from build123d import *

# Parameters (mm, degrees)
SKETCH1_R           = 65
SKETCH1_R_2         = 55
BOSS_EXTRUDE1_DEPTH = 250
BOSS_EXTRUDE2_START = 20
SKETCH3_R           = 55
SKETCH3_R_2         = 20
SKETCH3_R_3         = 13
BOSS_EXTRUDE2_DEPTH = 20
BOSS_EXTRUDE3_START = 210
SKETCH3_5_R         = 55
SKETCH3_5_R_2       = 20
SKETCH3_5_R_3       = 13
SKETCH3_5_R_4       = 6.5
BOSS_EXTRUDE3_DEPTH = 20
BOSS_EXTRUDE4_START = 20
SKETCH3_7_R         = 13
BOSS_EXTRUDE4_DEPTH = 210
SKETCH3_10_R        = 13
BOSS_EXTRUDE5_DEPTH = 20
BOSS_EXTRUDE6_START = 230
SKETCH3_11_R        = 13
BOSS_EXTRUDE6_DEPTH = 20


with BuildPart() as part:
    # Sketch1 → Boss-Extrude1 (new body)
    with BuildSketch(Plane(origin=(0, 0, 0), x_dir=(1, 0, 0), z_dir=(0, 1, 0))):
        with Locations(Location((0, 0, 0), (0, 0, 270))):
            Circle(SKETCH1_R)
        with Locations(Location((0, 0, 0), (0, 0, 270))):
            Circle(SKETCH1_R_2, mode=Mode.SUBTRACT)
    extrude(amount=BOSS_EXTRUDE1_DEPTH)

    # Sketch3 → Boss-Extrude2 (add)
    with BuildSketch(Plane(origin=(0, 0, 0), x_dir=(1, 0, 0), z_dir=(0, 1, 0)).offset(BOSS_EXTRUDE2_START)):
        with Locations(Location((0, 0, 0), (0, 0, 270))):
            Circle(SKETCH3_R)
        with BuildLine():
            ThreePointArc((39.298819185, 16.181866723), (42.375869887, 3.245866806), (41.304875194, -10.00786117))
            Line((41.304875194, -10.00786117), (19.437588327, -4.709581727))
            ThreePointArc((19.437588327, -4.709581727), (17.030904249, -10.485623513), (12.957116602, -15.235259412))
            Line((12.957116602, -15.235259412), (27.53387278, -32.374926251))
            ThreePointArc((27.53387278, -32.374926251), (16.181866723, -39.298819185), (3.245866806, -42.375869887))
            Line((3.245866806, -42.375869887), (1.527466732, -19.941585829))
            ThreePointArc((1.527466732, -19.941585829), (-4.709581727, -19.437588327), (-10.485623513, -17.030904249))
            Line((-10.485623513, -17.030904249), (-22.281949965, -36.190671529))
            ThreePointArc((-22.281949965, -36.190671529), (-32.374926251, -27.53387278), (-39.298819185, -16.181866723))
            Line((-39.298819185, -16.181866723), (-18.493561969, -7.614996105))
            ThreePointArc((-18.493561969, -7.614996105), (-19.941585829, -1.527466732), (-19.437588327, 4.709581727))
            Line((-19.437588327, 4.709581727), (-41.304875194, 10.00786117))
            ThreePointArc((-41.304875194, 10.00786117), (-36.190671529, 22.281949965), (-27.53387278, 32.374926251))
            Line((-27.53387278, 32.374926251), (-12.957116602, 15.235259412))
            ThreePointArc((-12.957116602, 15.235259412), (-7.614996105, 18.493561969), (-1.527466732, 19.941585829))
            Line((-1.527466732, 19.941585829), (-3.245866806, 42.375869887))
            ThreePointArc((-3.245866806, 42.375869887), (10.00786117, 41.304875194), (22.281949965, 36.190671529))
            Line((22.281949965, 36.190671529), (10.485623513, 17.030904249))
            ThreePointArc((10.485623513, 17.030904249), (15.235259412, 12.957116602), (18.493561969, 7.614996105))
            Line((18.493561969, 7.614996105), (39.298819185, 16.181866723))
        make_face(mode=Mode.SUBTRACT)
        Circle(SKETCH3_R_2)
        with Locations(Location((0, 0, 0), (0, 0, 270))):
            Circle(SKETCH3_R_3, mode=Mode.SUBTRACT)
    extrude(amount=BOSS_EXTRUDE2_DEPTH)

    # Sketch3_5 → Boss-Extrude3 (add)
    with BuildSketch(Plane(origin=(0, 0, 0), x_dir=(1, 0, 0), z_dir=(0, 1, 0)).offset(BOSS_EXTRUDE3_START)):
        with Locations(Location((0, 0, 0), (0, 0, 270))):
            Circle(SKETCH3_5_R)
        with BuildLine():
            ThreePointArc((39.298819185, 16.181866723), (42.375869887, 3.245866806), (41.304875194, -10.00786117))
            Line((41.304875194, -10.00786117), (19.437588327, -4.709581727))
            ThreePointArc((19.437588327, -4.709581727), (17.030904249, -10.485623513), (12.957116602, -15.235259412))
            Line((12.957116602, -15.235259412), (27.53387278, -32.374926251))
            ThreePointArc((27.53387278, -32.374926251), (16.181866723, -39.298819185), (3.245866806, -42.375869887))
            Line((3.245866806, -42.375869887), (1.527466732, -19.941585829))
            ThreePointArc((1.527466732, -19.941585829), (-4.709581727, -19.437588327), (-10.485623513, -17.030904249))
            Line((-10.485623513, -17.030904249), (-22.281949965, -36.190671529))
            ThreePointArc((-22.281949965, -36.190671529), (-32.374926251, -27.53387278), (-39.298819185, -16.181866723))
            Line((-39.298819185, -16.181866723), (-18.493561969, -7.614996105))
            ThreePointArc((-18.493561969, -7.614996105), (-19.941585829, -1.527466732), (-19.437588327, 4.709581727))
            Line((-19.437588327, 4.709581727), (-41.304875194, 10.00786117))
            ThreePointArc((-41.304875194, 10.00786117), (-36.190671529, 22.281949965), (-27.53387278, 32.374926251))
            Line((-27.53387278, 32.374926251), (-12.957116602, 15.235259412))
            ThreePointArc((-12.957116602, 15.235259412), (-7.614996105, 18.493561969), (-1.527466732, 19.941585829))
            Line((-1.527466732, 19.941585829), (-3.245866806, 42.375869887))
            ThreePointArc((-3.245866806, 42.375869887), (10.00786117, 41.304875194), (22.281949965, 36.190671529))
            Line((22.281949965, 36.190671529), (10.485623513, 17.030904249))
            ThreePointArc((10.485623513, 17.030904249), (15.235259412, 12.957116602), (18.493561969, 7.614996105))
            Line((18.493561969, 7.614996105), (39.298819185, 16.181866723))
        make_face(mode=Mode.SUBTRACT)
        Circle(SKETCH3_5_R_2)
        with Locations(Location((0, 0, 0), (0, 0, 270))):
            Circle(SKETCH3_5_R_3, mode=Mode.SUBTRACT)
        Circle(SKETCH3_5_R_4)
    extrude(amount=BOSS_EXTRUDE3_DEPTH)


with BuildPart() as boss_extrude3_kept_piece:
    # of the separate pieces the step leaves, the one the design keeps (boss_extrude3_pieces_kept)
    add(part.part.solids().sort_by_distance((0, 0, 65))[0])

    # Sketch3_7 → Boss-Extrude4 (add)
    with BuildSketch(Plane(origin=(0, 0, 0), x_dir=(1, 0, 0), z_dir=(0, 1, 0)).offset(BOSS_EXTRUDE4_START)):
        with Locations(Location((0, 0, 0), (0, 0, 270))):
            Circle(SKETCH3_7_R)
        with BuildLine():
            Line((2, 8.5), (2, 6.184658438))
            ThreePointArc((2, 6.184658438), (5.25594901, 3.824264635), (6.5, 0))
            ThreePointArc((6.5, 0), (-3.824264635, -5.25594901), (-2, 6.184658438))
            Line((-2, 6.184658438), (-2, 8.5))
            Line((-2, 8.5), (2, 8.5))
        make_face(mode=Mode.SUBTRACT)
        with BuildLine():
            ThreePointArc((-2, 6.184658438), (0, 6.5), (2, 6.184658438))
            Line((2, 6.184658438), (2, 8.5))
            Line((2, 8.5), (-2, 8.5))
            Line((-2, 8.5), (-2, 6.184658438))
        make_face()
    extrude(amount=BOSS_EXTRUDE4_DEPTH)

    # Sketch3_10 → Boss-Extrude5 (add)
    with BuildSketch(Plane(origin=(0, 0, 0), x_dir=(1, 0, 0), z_dir=(0, 1, 0))):
        with Locations(Location((0, 0, 0), (0, 0, 270))):
            Circle(SKETCH3_10_R)
        with BuildLine():
            Line((2, 5.656854249), (2, 8.5))
            Line((2, 8.5), (-2, 8.5))
            Line((-2, 8.5), (-2, 5.656854249))
            ThreePointArc((-2, 5.656854249), (0, -6), (2, 5.656854249))
        make_face(mode=Mode.SUBTRACT)
    extrude(amount=BOSS_EXTRUDE5_DEPTH)

    # Sketch3_11 → Boss-Extrude6 (add)
    with BuildSketch(Plane(origin=(0, 0, 0), x_dir=(1, 0, 0), z_dir=(0, 1, 0)).offset(BOSS_EXTRUDE6_START)):
        with Locations(Location((0, 0, 0), (0, 0, 270))):
            Circle(SKETCH3_11_R)
        with BuildLine():
            Line((2, 5.656854249), (2, 8.5))
            Line((2, 8.5), (-2, 8.5))
            Line((-2, 8.5), (-2, 5.656854249))
            ThreePointArc((-2, 5.656854249), (0, -6), (2, 5.656854249))
        make_face(mode=Mode.SUBTRACT)
    extrude(amount=BOSS_EXTRUDE6_DEPTH)


solid = boss_extrude3_kept_piece.part
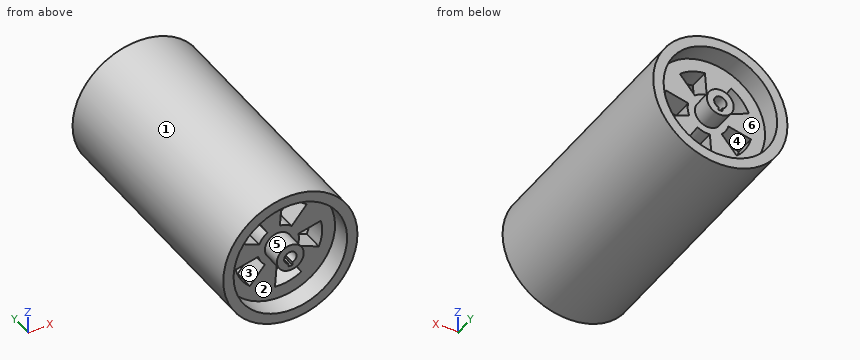
Model file for the job. Use its own axes, mm. Face numbers are marked on the shaded views. A direction names the side the tool comes from. Give positions to 0.01 mm unless a question says otherwise; leave off trailing zeros. Write each loop counter-clockwise with the first axis right and the second up, starting at its lowest first coordinate (ties: lowest second). Pieces come first, ordered by that corner, then holes. Notation, with made-up numbers: M 75,-18.5 L 130,-18.5 A23 ccw 130,7.5 Z; hole C -12.5,28.25 d10. An arc over 180 degrees is marked long. One line per item, written item: value. Start each with the question number.
Q1. Saw through at A-A, the plane y = 217.5. Write the cut outline in (x, z) (3 decimals), plus the area to 3 significant figures.
Q2. Probe probe 1 along X at (y, z) = (19, 0); probe 2 along Y at (x, z) = (39, -35.5); probe 3 along X at (y, z) = (146.5, 4.5). List the from-to ranges inside material, lowest first. Write a range as [from, to].
Q3. Saw through at B-B, the plane z = -23. State how many separate pieces and enclosed holes the cut face has, plus the area to 3 significant figures.
Q4. Drop flat-ended pins along their axis: pin 1 Ø3 at (y, z) = (238.5, -7.5) entering from -X; pin 2 Ø4 at (y, z) = (42, 25) entering from +X; pin 3 Ø2 at (x, y) = (-0.5, 235.5) entering from +Z; pin 4 Ø1 at (x, z) = (-20, 4.5) entering from -Y. Give the stop position or say it passes through.
Q5. Saw through at C-C, the plane y = 147. Write the cut outline in (x, z).
Q6. 3-axis set-ups, long thin cutter, end or side, ignore diameter. For the marked faces 4, 5 and 6: which of +Z, -Z, +X, -X, +Y, -Y reach the whole face in a straight line?
Q7. Two-plate mould, pull along X, no slides. Class the marked faces 1, 2 and 3: +X half, -X half, draft (parallel to the pull), parting line (faces both ways), or undercut.
Output values:
1. outline: C 0,0 d130; hole M -41.305,-10.008 A42.5 ccw -27.534,-32.375 L -12.957,-15.235 A20 cw -19.438,-4.71 Z; hole M -39.299,16.182 L -18.494,7.615 A20 cw -10.486,17.031 L -22.282,36.191 A42.5 ccw Z; hole C 0,0 d13; hole M -3.246,-42.376 A42.5 ccw 22.282,-36.191 L 10.486,-17.031 A20 cw -1.527,-19.942 Z; hole M 1.527,19.942 A20 cw 12.957,15.235 L 27.534,32.375 A42.5 ccw 3.246,42.376 Z; hole M 18.494,-7.615 L 39.299,-16.182 A42.5 ccw 41.305,10.008 L 19.438,4.71 A20 cw Z
1. area: 10,900 mm²
2. probe 1: x = [-65, -55], [-13, -6], [6, 13], [55, 65]
2. probe 2: y = [20, 40], [210, 230]
2. probe 3: x = [-64.84, -54.82], [-12.2, -4.69], [4.69, 12.2], [54.82, 64.84]
3. separate pieces: 4
3. enclosed holes: 0
3. area: 8,130 mm²
4. pin 1: stops at x = -64.72
4. pin 2: stops at x = 60.79
4. pin 3: stops at z = 65
4. pin 4: stops at y = 20
5. outline: C 0,0 d130; C 0,0 d26; hole C 0,0 d110; hole C 0,0 d13
6. face 4: +Y, -Y
6. face 5: -Y
6. face 6: +Y
7. face 1: parting line
7. face 2: undercut
7. face 3: undercut
